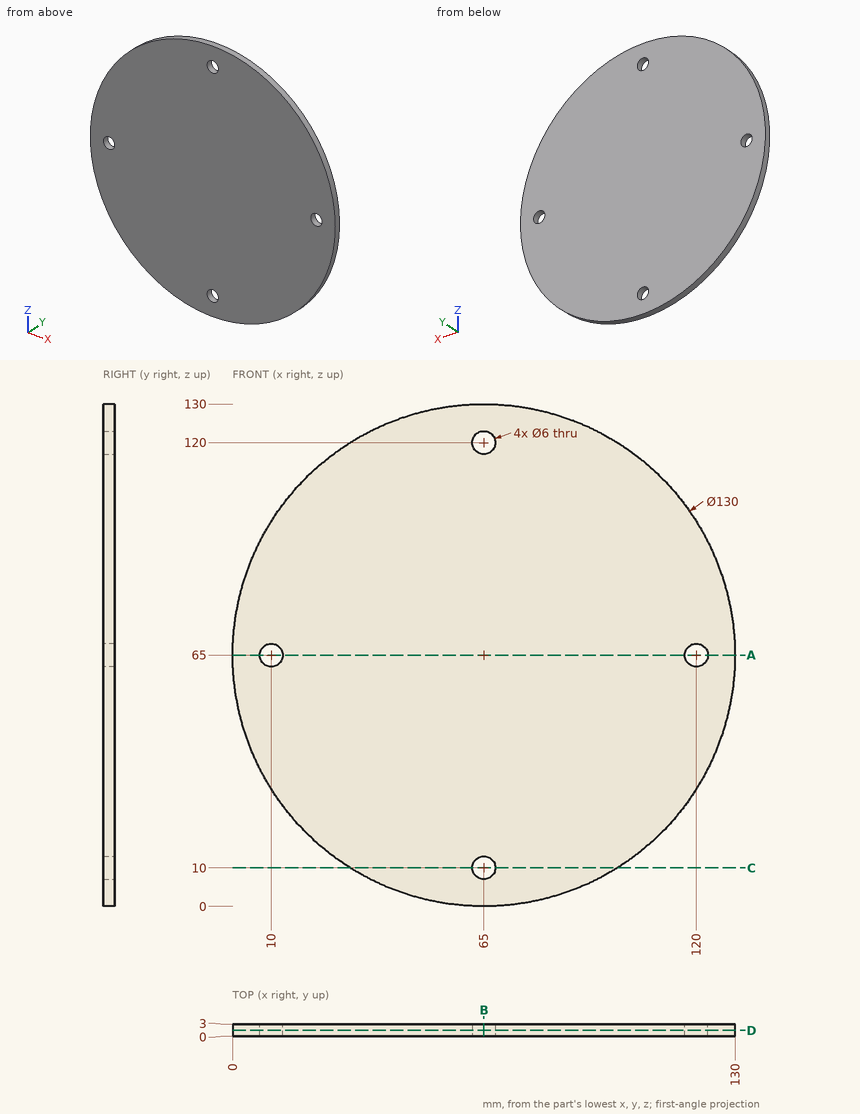
Source: three-view drawing plus pictorial views. Frame: mm from the lowest corner of the part. Round coordinates to 2 decimals unless told otherwise and drop trailing zeros. Loops run counter-clockwise (first coordinate to the right, second up) from the corner with the lowest first, then second, coordinate; pieces in that order, holes last. Notation, with made-up numbers: M 47,76 L 79,76 A32 ccw 79,103 Z; hole C 76.25,75.25 d1. An arc over 180 degrees is marked long. Put each result on its own line as item: value.
(1) Section C-C, the plane z = 10. Return loops of the section in (x, y).
Solutions:
outline: M 30.36,0 L 62,0 L 62,3 L 30.36,3 Z; M 68,0 L 99.64,0 L 99.64,3 L 68,3 Z
(2) Section A-A, the plane z = 65. Return loops of the section in (x, y).
Solutions:
outline: M 0,0 L 7,0 L 7,3 L 0,3 Z; M 13,0 L 117,0 L 117,3 L 13,3 Z; M 123,0 L 130,0 L 130,3 L 123,3 Z
(3) Ray query, line 1 (X direction, y = 1.4, z = 65); line 2 (Z direction, x = 63.5, y = 1.75). Return the intervals inside material, ascending. Write a range as [from, to].
Solutions:
line 1: [0, 7], [13, 117], [123, 130]
line 2: [0.02, 7.4], [12.6, 117.4], [122.6, 129.98]
(4) First-contact query: pin 1 (5 mm diameter, centred on x = 10, z = 65, fed in from -Y). Flat tip, straight axial feed; report the tip coordinate or a pass-through.
Solutions:
pin 1: through
(5) Section D-D, the plane y = 1.45. Return loops of the section in (x, z), and give its area (3 significant figures).
Solutions:
outline: C 65,65 d130; hole C 10,65 d6; hole C 65,10 d6; hole C 65,120 d6; hole C 120,65 d6
area: 13,200 mm²
(6) Section B-B, the plane x = 65. Return loops of the section in (y, z), and give its area (3 significant figures).
Solutions:
outline: M 0,0 L 3,0 L 3,7 L 0,7 Z; M 0,13 L 3,13 L 3,117 L 0,117 Z; M 0,123 L 3,123 L 3,130 L 0,130 Z
area: 354 mm²
